Can you work these out from the model? Positions are in its coordinate system, mm. Face numbers are marked on the shaded views. A direction names the side the tool comes from. Coordinates: 2 decimals unless noted, no trailing zeros. Write each loop counter-clockwise with the first axis right and the second up, starting at its lowest first coordinate (ties: lowest second). Pieces come first, ordered by that corner, then holes. Notation, with made-up numbers: (-9.5, -30) - (3.5, -30) arc R35 ccw to (3.5, 2) - close; hole circle Ø9 at (-40, 12.5). An arc over 180 degrees is marked (long way). One line per question, with ' | ' between items. Start each with the question number.
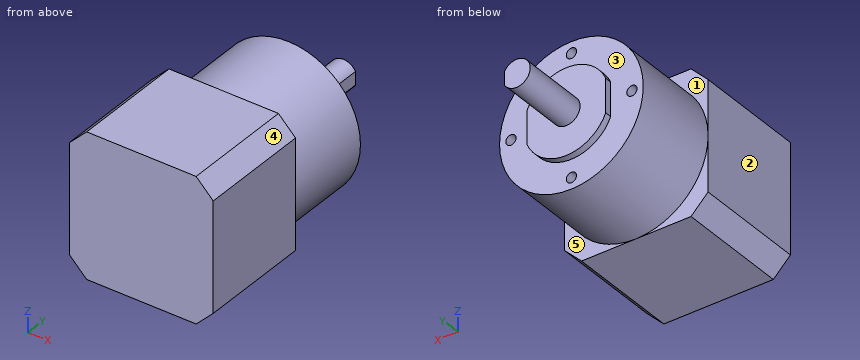
Autodesk Inventor part; units mm, degrees
ref_plane "YZ Plane" through (0, 0, 0) normal (1, 0, 0) x (0, 1, 0)
ref_plane "XZ Plane" through (0, 0, 0) normal (0, 1, 0) x (-1, 0, 0)
ref_plane "XY Plane" through (0, 0, 0) normal (0, 0, 1) x (1, 0, 0)
sketch "Sketch1" plane through (0, 0, 0) normal (0, 1, 0) x (-1, 0, 0)
  line L0 (0, 0) -> (0, -42)
  line L1 (0, -42) -> (42, -42)
  line L2 (42, -42) -> (42, 0)
  line L3 (42, 0) -> (0, 0)
  dimension "d0" = 42
  dimension "d1" = 42
extrude "Extrusion1" add sketch "Sketch1" along normal blind 33
chamfer "Chamfer1" distance 5 angle 45 4 edges at (0, 16.5, 0) (-42, 16.5, 0) (-42, 16.5, -42) (0, 16.5, -42)
sketch "Sketch2" plane through (0, 33, 0) normal (0, 1, 0) x (1, 0, 0)
  line L0 (-5, 42) -> (-37, 42)
  line L1 (0, 5) -> (0, 37)
  circle A0 centre (-21, 21) radius 21
  point P0 (0, 0)
  dimension "d7" = 42
  dimension "d8" = 21
  dimension "d9" = 21
extrude "Extrusion2" add sketch "Sketch2" along normal blind 26
sketch "Sketch3" plane through (-21, 59, -21) normal (0, 1, 0) x (1, 0, 0)
  circle A0 centre (0, 0) radius 21
  line L0 (11.5, 4.899) -> (11.5, -4.899)
  line L1 (-11.5, 4.899) -> (-11.5, -4.899)
  arc A1 (-11.5, -4.899) -> (11.5, -4.899) centre (0, 0) ccw
  arc A2 (11.5, 4.899) -> (-11.5, 4.899) centre (0, 0) ccw
  point P0 (21, -21)
  dimension "d13" = 11.5
  dimension "d14" = 11.5
  dimension "d15" = 12.5
  dimension "d16" = 12.5
extrude "Extrusion3" add sketch "Sketch3" along normal blind 2 contours L0 A1 L1 A2
sketch "Sketch4" plane through (-21, 61, -21) normal (0, 1, 0) x (1, 0, 0)
  arc A0 (11.5, 4.899) -> (-11.5, 4.899) centre (0, 0) ccw
  arc A1 (-11.5, -4.899) -> (11.5, -4.899) centre (0, 0) ccw
  arc A2 (3.5, 1.9365) -> (3.5, -1.9365) centre (0, 0) ccw
  line L0 (3.5, 1.9365) -> (3.5, -1.9365)
  point P0 (21, -21)
  dimension "d19" = 8
  dimension "d20" = 3.5
extrude "Extrusion4" add sketch "Sketch4" along normal blind 20
sketch "Sketch5" plane through (-21, 59, -21) normal (0, 1, 0) x (1, 0, 0)
  arc A0 (-11.5, -4.899) -> (11.5, -4.899) centre (0, 0) ccw
  circle A1 centre (0, -17.6777) radius 1.5
  circle A2 centre (17.6777, 0) radius 1.5
  circle A3 centre (0, 17.6777) radius 1.5
  circle A4 centre (-17.6777, 0) radius 1.5
  point P0 (21, -21)
  dimension "d23" = 3
  dimension "d26" = 25
  dimension "d27" = 25
  dimension "d29" = 17.6777
  dimension "d30" = 17.6777
  dimension "d31" = 17.6777
  dimension "d32" = 17.6777
extrude "Extrusion5" cut sketch "Sketch5" against normal blind 9
thread "Thread1"
thread "Thread2"
thread "Thread3"
thread "Thread4"
equation "\"d30\" = d29"
equation "\"d32\" = d31"
properties part number "StepperMotorNema17Geared" material "Aluminum 6061"
(1) If we section it at C-C on x = -10.5: List the corners of the cut face in (y, z) for me.
(2) If we section it at B-B on z = -27: List the corners of the cut face in (x, y) for me.
(3) If I drill on probe 1 along Z at (x, y) = (-21, 54); probe 2 along Y at (x, z) = (-2, -24.5), over which ranges is the centre line in solid material (lowest first)?
(4) I'm going to push flat-ended pins straight in: pin 1 (1 mm diameter, centred on y = 60.5, z = -19.5, fed in from +X); pin 2 (3.5 mm diameter, centred on x = -3.32, z = -21, fed in from +Y); pin 3 (12.5 mm diameter, centred on x = -14, z = -16.5, fed in from +Y); pin 4 (8 mm diameter, centred on y = 40.5, z = -29.5, fed in from -X). Where does each tip first touch, or does it pass through?
(5) Which directions (+Z, -Z, +X, -X, +Y, -Y) give clear straight access to the entire face, cutting with the end or side of a thin tool? Please do the marked faces 1, 2, 3, 4 and 5.
(6) If we section it at D-D on y = 75: List the corners of the cut face in (x, z) for me, plus the area to 3 significant figures.
(7) If we section it at A-A on y = 7.5: List the corners of the cut face in (x, z) for me, plus the area to 3 significant figures.
Values:
1) outline: (0, -42) - (33, -42) - (33, -39.19) - (59, -39.19) - (59, -27.78) - (61, -27.78) - (61, -14.22) - (59, -14.22) - (59, -2.81) - (33, -2.81) - (33, 0) - (0, 0) - close
2) outline: (-42, 0) - (0, 0) - (0, 33) - (-0.88, 33) - (-0.88, 59) - (-10.03, 59) - (-10.03, 61) - (-31.97, 61) - (-31.97, 59) - (-41.12, 59) - (-41.12, 33) - (-42, 33) - close
3) probe 1: -42 to -40.18, -37.18 to -4.82, -1.82 to 0 | probe 2: 0 to 59
4) pin 1: x = -9.5 | pin 2: y = 59 | pin 3: y = 81 | pin 4: x = -41.51
5) face 1: +Z, -X, +Y | face 2: +Z, -Z, -X, +Y, -Y | face 3: +Y | face 4: +Z, +X, +Y, -Y | face 5: -Z, +X, +Y
6) outline: (-17.5, -22.94) - (-17.5, -19.06) arc R4 ccw (long way) to start | area: 49.0 mm2
7) outline: (-42, -37) - (-37, -42) - (-5, -42) - (0, -37) - (0, -5) - (-5, 0) - (-37, 0) - (-42, -5) - close | area: 1,710 mm2
